Autodesk Fusion 360 part; units mm, degrees
sketch "Sketch1" plane through (0, 0, 0) normal (0, 1, 0) x (1, 0, 0)
  line L0 (0, 0) -> (200, 0)
  line L1 (200, 0) -> (200, -150)
  line L2 (200, -150) -> (0, -150)
  line L3 (0, -150) -> (0, 0)
  dimension "d1" = 200
  dimension "d2" = 150
extrude "Extrude1" add sketch "Sketch1" along normal blind 2
sketch "Sketch2" plane through (0, 0, 0) normal (0, -1, 0) x (1, 0, 0)
  line L0 (200, 150) -> (0, 150)
  line L1 (0, 150) -> (0, 0)
  line L2 (0, 0) -> (200, 0)
  line L3 (200, 0) -> (200, 150)
  line L4 (4, 112.5) -> (35, 112.5)
  line L5 (35, 112.5) -> (35, 115.5)
  line L6 (35, 115.5) -> (4, 115.5)
  line L7 (4, 115.5) -> (4, 112.5)
  line L8 (37, 117.5) -> (2, 117.5)
  line L9 (2, 117.5) -> (2, 110.5)
  line L10 (2, 110.5) -> (37, 110.5)
  line L11 (37, 110.5) -> (37, 117.5)
  line L12 (200, 150) -> (0, 150)
  line L13 (0, 150) -> (0, 0)
  line L14 (0, 0) -> (200, 0)
  line L15 (200, 0) -> (200, 150)
  line L16 (2, 110.5) -> (37, 110.5)
  line L17 (200, 150) -> (0, 150)
  line L18 (0, 150) -> (0, 0)
  line L19 (0, 150) -> (0, 0)
  line L20 (35, 37.5) -> (35, 34.5)
  line L21 (0, 0) -> (200, 0)
  line L22 (122, 39.5) -> (157, 39.5)
  line L23 (35, 112.5) -> (35, 115.5)
  line L24 (37, 110.5) -> (2, 110.5)
  line L25 (2, 110.5) -> (2, 117.5)
  line L26 (2, 117.5) -> (37, 117.5)
  line L27 (37, 117.5) -> (37, 110.5)
  dimension "d5" = 31
  dimension "d6" = 3
  dimension "d7" = 35
  dimension "d8" = 7
  dimension "d9" = 2
  dimension "d10" = 2
  dimension "d18" = 32.5
  dimension "d19" = 2
extrude "Extrude2" add sketch "Sketch2" along normal blind 10 contours L8 L9 L10 L11 L16 L24 L25 L26 L27
sketch "Sketch3" plane through (0, 0, 0) normal (0, -1, 0) x (1, 0, 0)
  line L0 (200, 150) -> (0, 150)
  line L1 (0, 150) -> (0, 0)
  line L2 (0, 0) -> (200, 0)
  line L3 (200, 0) -> (200, 150)
  line L4 (4, 37.5) -> (35, 37.5)
  line L5 (35, 37.5) -> (35, 34.5)
  line L6 (35, 34.5) -> (4, 34.5)
  line L7 (4, 34.5) -> (4, 37.5)
  line L8 (2, 39.5) -> (37, 39.5)
  line L9 (37, 39.5) -> (37, 32.5)
  line L10 (37, 32.5) -> (2, 32.5)
  line L11 (2, 32.5) -> (2, 39.5)
  line L12 (2, 110.5) -> (37, 110.5)
  line L13 (0, 150) -> (0, 0)
  line L14 (37, 110.5) -> (2, 110.5)
  line L15 (2, 110.5) -> (2, 117.5)
  line L16 (2, 117.5) -> (37, 117.5)
  line L17 (37, 117.5) -> (37, 110.5)
  dimension "d11" = 3
  dimension "d12" = 31
  dimension "d13" = 2
  dimension "d14" = 7
  dimension "d15" = 35
  dimension "d16" = 2
  dimension "d17" = 71
  dimension "d20" = 2
extrude "Extrude3" add sketch "Sketch3" along normal blind 10 contours L8 L9 L10 L11
sketch "Sketch4" plane through (0, 0, 0) normal (0, -1, 0) x (1, 0, 0)
  line L0 (124, 37.5) -> (155, 37.5)
  line L1 (155, 37.5) -> (155, 34.5)
  line L2 (155, 34.5) -> (124, 34.5)
  line L3 (124, 34.5) -> (124, 37.5)
  line L4 (122, 39.5) -> (157, 39.5)
  line L5 (157, 39.5) -> (157, 32.5)
  line L6 (157, 32.5) -> (122, 32.5)
  line L7 (122, 32.5) -> (122, 39.5)
  line L8 (35, 37.5) -> (35, 34.5)
  line L9 (0, 0) -> (200, 0)
  dimension "d21" = 31
  dimension "d22" = 3
  dimension "d23" = 35
  dimension "d24" = 7
  dimension "d25" = 2
  dimension "d26" = 2
  dimension "d28" = 89
  dimension "d29" = 32.5
sketch "Sketch5" plane through (0, 0, 0) normal (0, -1, 0) x (1, 0, 0)
  line L0 (124, 115.5) -> (155, 115.5)
  line L1 (155, 115.5) -> (155, 112.5)
  line L2 (155, 112.5) -> (124, 112.5)
  line L3 (124, 112.5) -> (124, 115.5)
  line L4 (122, 117.5) -> (157, 117.5)
  line L5 (157, 117.5) -> (157, 110.5)
  line L6 (157, 110.5) -> (122, 110.5)
  line L7 (122, 110.5) -> (122, 117.5)
  line L8 (122, 39.5) -> (157, 39.5)
  line L9 (35, 112.5) -> (35, 115.5)
  dimension "d30" = 31
  dimension "d31" = 3
  dimension "d32" = 35
  dimension "d33" = 7
  dimension "d35" = 2
  dimension "d36" = 2
  dimension "d37" = 71
  dimension "d38" = 89
extrude "Extrude4" add sketch "Sketch4" along normal blind 10
extrude "Extrude5" add sketch "Sketch5" along normal blind 10
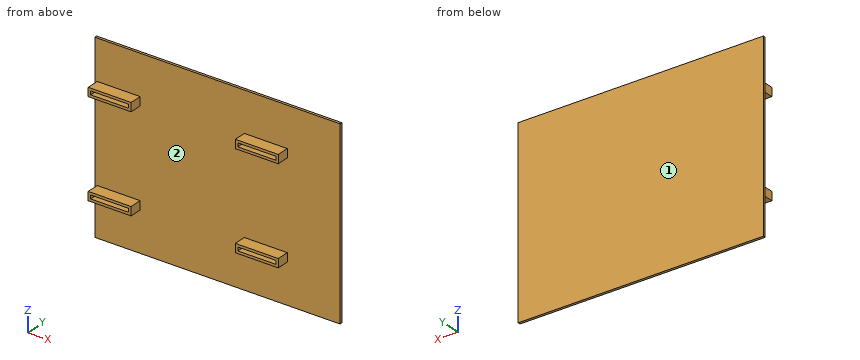
Build history of the part. All positions in model axes, mm. Face numbers are marked on the shaded views. Coordinates: 2 decimals unless noted, no trailing zeros. Order: outer loops, then holes, each group sorted by start corner. A loop starts at its lowest first (then second) coordinate and runs counter-clockwise, first axis right, second up. Notation, with made-up numbers: (60, 50.25) - (82, 50.25) arc R8 cw to (82, 58.25) - close; hole circle Ø2 at (-20.5, -4.5). An arc over 180 degrees is marked (long way). Write each question's results on one line, items separated by ' | '. Start each with the question number.
Item 1: Wall check: probe 1 along Z at (x, y) = (26.5, -5.5); probe 2 along Y at (x, z) = (160, 25). Give the ranges that are in metal, low to high. Write a range as [from, to].
Item 2: Band-saw the part on A-A on y = -2.25. State how many separate pieces and enclosed holes the cut face has, and give its area (3 significant figures).
Item 3: Band-saw the part on C-C on x = 117.5. Write the cut outline in (y, z), and give its area (3 significant figures).
Item 4: Mould opens along Z. For the marked faces 1 and 2 say: released by +Z, released by -Z, zero draft, split by the parting line, or undercut.
Item 5: Flat gauge pins, fed straight in: pin 1 (3 mm diameter, centred on x = 19.5, y = -5, fed in from -Z); pin 2 (5.5 mm diameter, centred on y = -3.5, z = 113, fed in from -X); pin 3 (1.5 mm diameter, centred on y = -2.5, z = 35.5, fed in from +X). Where does each tip first touch, or does it go through?
Item 6: Band-saw the part on B-B on z = 126.5. Write the cut outline in (x, y), and give its area (3 significant figures).
Numbers:
1) probe 1: [32.5, 34.5], [37.5, 39.5], [110.5, 112.5], [115.5, 117.5] | probe 2: [0, 2]
2) separate pieces: 4 | enclosed holes: 4 | area: 608 mm^2
3) outline: (0, 0) - (2, 0) - (2, 150) - (0, 150) - close | area: 300 mm^2
4) face 1: zero draft | face 2: undercut
5) pin 1: z = 32.5 | pin 2: x = 2 | pin 3: x = 157
6) outline: (0, 0) - (200, 0) - (200, 2) - (0, 2) - close | area: 400 mm^2
